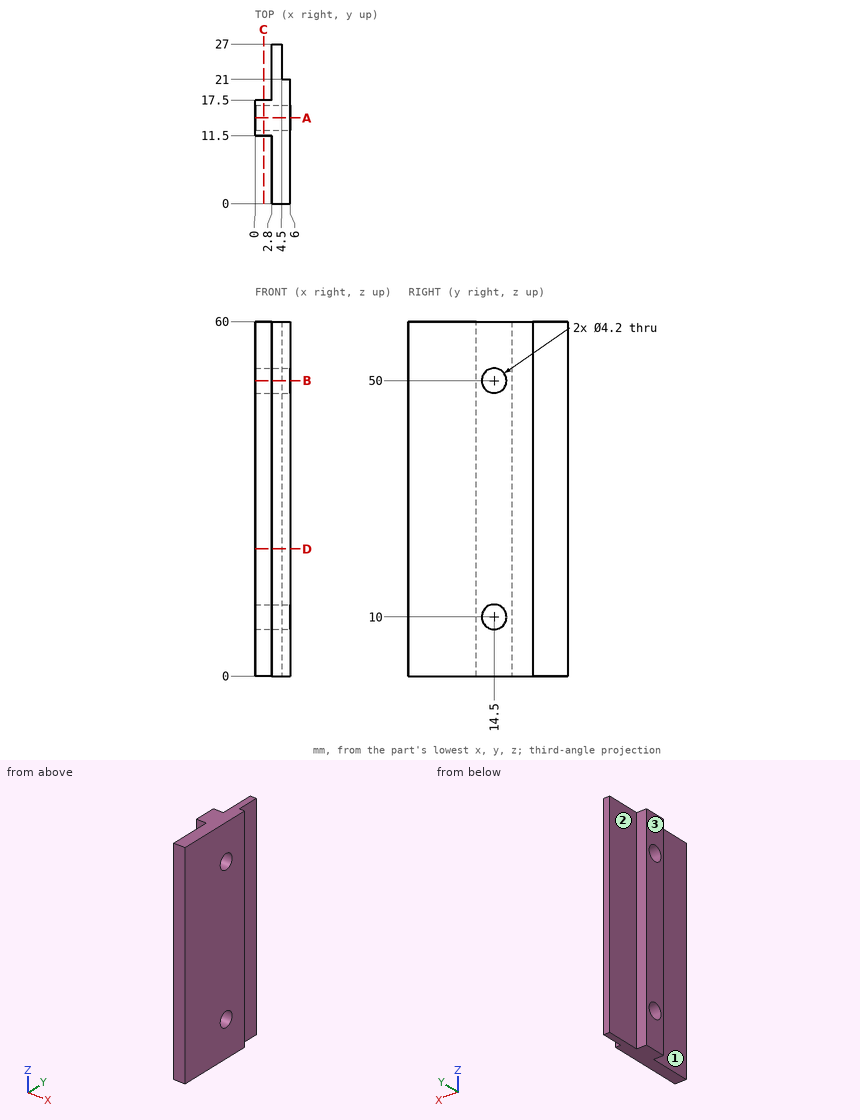
Answer from the drawing. Dimensions are ordinates in mm from the lowest x, y and z of the part. A direction names the side the tool comes from. Give positions to 0.01 mm unless a question says otherwise; leave off trailing zeros. Loops run counter-clockwise (first coordinate to the right, second up) from the corner with the lowest first, then second, coordinate; pieces in that order, holes last. Notation, with made-up numbers: (-19, 81.25) - (40, 81.25) arc R9 ccw to (40, 97.25) - close; hole circle Ø10 at (39.25, 86). An arc over 180 degrees is marked (long way). Answer as CSV lines item,"result". Start each with the question number.
Item 1: A cutting plane is placed at B-B on z = 50. Determine the outline of the cut face in (x, y).
Item 2: A cutting plane is placed at A-A on y = 14.5. Determine the outline of the cut face in (x, z), then the cut area to 3 significant figures.
Item 3: A cutting plane is placed at D-D on z = 21.5. Determine the outline of the cut face in (x, y).
Item 4: Find the intervals of material crossed by line 1 (Z direction, x = 2.2, y = 14.5); line 2 (Y direction, x = 1.35, z = 10); line 3 (Y direction, x = 4, z = 10), in increasing order. Write a range as from..to.
Item 5: For the marked faces 1, 2 and 3, determine the directions among +Z, -Z, +X, -X, +Y, -Y from which every point of the face is accessible in a straight line to the end or side of a thin tool.
Item 6: Each of these flat-tipped pins is pushed along its axis until it touches: pin 1 (1.6 mm diameter, centred on x = 5, z = 32, fed in from +Y); pin 2 (1.8 mm diameter, centred on y = 23, z = 44, fed in from +X); pin 3 (3 mm diameter, centred on x = 1, z = 25.5, fed in from +Y). Where does it stop, or does it pass through?
Item 7: A cutting plane is placed at C-C on x = 1.45. Determine the outline of the cut face in (y, z), then the cut area to 3 significant figures.
Found:
1,outline,"(0, 11.5) - (2.8, 11.5) - (2.8, 0) - (6, 0) - (6, 12.4) - (0, 12.4) - close; (0, 16.6) - (6, 16.6) - (6, 21) - (4.5, 21) - (4.5, 27) - (2.8, 27) - (2.8, 17.5) - (0, 17.5) - close"
2,outline,"(0, 0) - (6, 0) - (6, 7.9) - (0, 7.9) - close; (0, 12.1) - (6, 12.1) - (6, 47.9) - (0, 47.9) - close; (0, 52.1) - (6, 52.1) - (6, 60) - (0, 60) - close"
2,area,"310 mm^2"
3,outline,"(0, 11.5) - (2.8, 11.5) - (2.8, 0) - (6, 0) - (6, 21) - (4.5, 21) - (4.5, 27) - (2.8, 27) - (2.8, 17.5) - (0, 17.5) - close"
4,line 1,"z = 0..7.9, 12.1..47.9, 52.1..60"
4,line 2,"y = 11.5..12.4, 16.6..17.5"
4,line 3,"y = 0..12.4, 16.6..27"
5,face 1,"+Z, -Z, -X, -Y"
5,face 2,"+Z, -Z, -X, +Y"
5,face 3,"+Z, -Z, -X, +Y, -Y"
6,pin 1,"stops at y = 27"
6,pin 2,"stops at x = 4.5"
6,pin 3,"stops at y = 17.5"
7,outline,"(11.5, 0) - (17.5, 0) - (17.5, 60) - (11.5, 60) - close; hole circle Ø4.2 at (14.5, 10); hole circle Ø4.2 at (14.5, 50)"
7,area,"332 mm^2"
